from build123d import *

# Parameters (mm, degrees)
BOSS_EXTRUDE1_DEPTH                               = 3.175
FILLET1_R                                         = 6.35
CSK_FOR_6_FLAT_HEAD_MACHINE_SCREW_100_D           = 4.3053
CSK_FOR_6_FLAT_HEAD_MACHINE_SCREW_100_CSINK_D     = 7.0866
CSK_FOR_6_FLAT_HEAD_MACHINE_SCREW_100_CSINK_ANGLE = 100
CSK_FOR_8_FLAT_HEAD_MACHINE_SCREW_2_COUNT         = 2
CSK_FOR_8_FLAT_HEAD_MACHINE_SCREW_2_PITCH         = 22.895250599
CHAMFER1_SIZE                                     = 2.54


with BuildPart() as part:
    # Sketch1 → Boss-Extrude1 (new body)
    with BuildSketch(Plane.ZY.offset(-5.035827965)):
        Polygon((-147.77562455, 230.070458845), (-159.314588786, 295.511176933), (-159.314588786, 330.563176933), (-120.626834873, 330.563176933), (-120.626834873, 295.511176933), (-110.25444916, 236.686454414), align=None)
    extrude(amount=BOSS_EXTRUDE1_DEPTH)

    # Fillet1
    fillet1_edges = [part.edges().sort_by_distance(p)[0] for p in [
        (3.448327965, 295.511176933, -159.314588786),
        (3.448327965, 295.511176933, -120.626834873),
    ]]
    fillet(fillet1_edges, radius=FILLET1_R)

    # CSK for #6 Flat Head Machine Screw (100)1 (through all)
    with Locations(Plane.ZY.offset(-1.860827965)):
        with Locations((-124.504125043, 273.139415456), (-144.485224025, 269.724179148), (-140.075144867, 244.324179148), (-120.227402214, 247.716621746)):
            CounterSinkHole(CSK_FOR_6_FLAT_HEAD_MACHINE_SCREW_100_D / 2, CSK_FOR_6_FLAT_HEAD_MACHINE_SCREW_100_CSINK_D / 2, counter_sink_angle=CSK_FOR_6_FLAT_HEAD_MACHINE_SCREW_100_CSINK_ANGLE)

    # Sketch5 → CSK for #8 Flat Head Machine Screw (100)1 (revolve, cut)
    with BuildSketch(Plane(origin=(1.860827965, 320.911176933, -149.328834873), x_dir=(0, 0, 1), z_dir=(0, 1, 0))):
        Polygon((0, 0), (0, 3.175), (2.45745, 3.175), (2.45745, 1.475934296), (4.2164, 0), align=None)
    csk_for_8_flat_head_machine_screw_100 = revolve(axis=Axis((-4.489172035, 320.911176933, -149.328834873), (1, 0, 0)), mode=Mode.SUBTRACT)

    # CSK for _8 Flat Head Machine Screw _ 2: CSK for #8 Flat Head Machine Screw (100)1 ×2
    with Locations(*[Vector(0, -0.554700196, 0.832050294) * (i * CSK_FOR_8_FLAT_HEAD_MACHINE_SCREW_2_PITCH) for i in range(1, CSK_FOR_8_FLAT_HEAD_MACHINE_SCREW_2_COUNT)]):
        add(csk_for_8_flat_head_machine_screw_100, mode=Mode.SUBTRACT)

    # Chamfer1
    chamfer1_edges = [part.edges().sort_by_distance(p)[0] for p in [
        (3.448327965, 230.070458845, -147.77562455),
        (3.448327965, 330.563176933, -159.314588786),
        (3.448327965, 330.563176933, -120.626834873),
        (3.448327965, 236.686454414, -110.25444916),
    ]]
    chamfer(chamfer1_edges, length=CHAMFER1_SIZE)


solid = part.part
Here's how the part is built. I have some questions about the finished solid (model axes, mm). Coordinates: 2 decimals unless noted, no trailing zeros. Order: outer loops, then holes, each group sorted by start corner. A loop starts at its lowest first (then second) coordinate and runs counter-clockwise, first axis right, second up. Notation, with made-up numbers: (86.25, 41.25) -> (95.25, 41.25) arc R12 ccw to (95.25, 58.25) -> close; hole circle Ø3 at (-15.5, -25.75). An arc over 180 degrees is marked (long way). Answer in a Markdown table with one row per item.
(1) Thinking about a two-plate mould opening in Z: for faces 1 (the face through (3, 312, -159.315)), 2 (the face through (4.174, 318.475, -149.649)), 3 (the face through (1.861, 281, -135)), which applies, +Z half, -Z half, draft (parallel to the pull), parting line (faces both ways), or undercut?
Answer key:
| item | result |
|---|---|
| face 1 | -Z half |
| face 2 | undercut |
| face 3 | draft |
(2) I want a section at C-C on z = -155. List the corners of the cut face in (x, y) for me.
Answer key:
| item | result |
|---|---|
| outline | (1.86, 271.04) -> (5.04, 271.04) -> (5.04, 330.56) -> (1.86, 330.56) -> close |
(3) Please list where these lines run through material, in increasing order: probe 1 along Z at (x, y) = (2.15, 271.5); probe 2 along Z at (x, y) = (3.4, 303); probe 3 along Z at (x, y) = (2.8, 322.5).
Answer key:
| item | result |
|---|---|
| probe 1 | -155.08 to -147.15, -141.82 to -127.25, -121.76 to -116.39 |
| probe 2 | -159.31 to -120.63 |
| probe 3 | -159.31 to -151.99, -146.67 to -120.63 |
(4) Will these pins go through, and if not, where does the flat tip stop? pin 1 Ø5 at (y, z) = (247.72, -120.23) entering from -X; pin 2 Ø8 at (y, z) = (308.21, -130.28) entering from -X; pin 3 Ø2.5 at (y, z) = (244.32, -140.08) entering from +X; pin 4 Ø5.5 at (y, z) = (273.14, -124.5) entering from -X.
Answer key:
| item | result |
|---|---|
| pin 1 | x = 2.73 |
| pin 2 | x = 2.04 |
| pin 3 | through |
| pin 4 | x = 2.52 |
(5) I want a section at A-A on x = 2.5. List the corners of the cut face in (y, z) for me.
Answer key:
| item | result |
|---|---|
| outline | (230.51, -145.27) -> (232.57, -148.22) -> (294.96, -159.22) arc R6.35 ccw to (296.07, -159.31) -> (328.02, -159.31) -> (330.56, -156.77) -> (330.56, -123.17) -> (328.02, -120.63) -> (296.07, -120.63) arc R6.35 cw to (294.96, -120.53) -> (239.19, -110.7) -> (236.25, -112.76) -> close; hole circle Ø5.56 at (244.32, -140.08); hole circle Ø5.56 at (247.72, -120.23); hole circle Ø5.56 at (269.72, -144.49); hole circle Ø5.56 at (273.14, -124.5); hole circle Ø6.91 at (308.21, -130.28); hole circle Ø6.91 at (320.91, -149.33) |
(6) I want a section at B-B on y = 286. List the corners of the cut face in (x, z) for me.
Answer key:
| item | result |
|---|---|
| outline | (1.86, -157.64) -> (5.04, -157.64) -> (5.04, -118.95) -> (1.86, -118.95) -> close |
